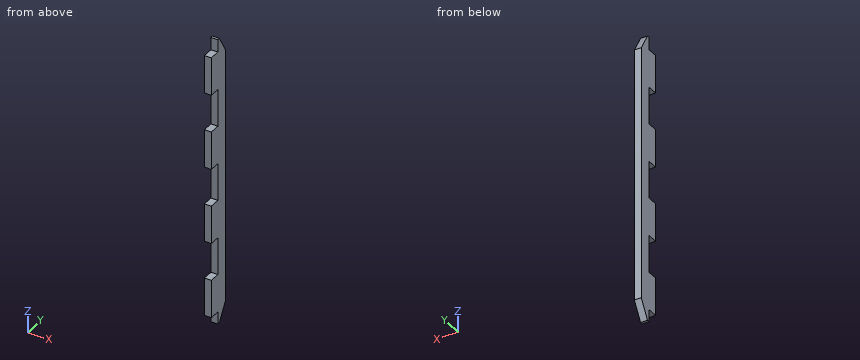
Autodesk Inventor part; units mm, degrees
ref_plane "YZ Plane" through (0, 0, 0) normal (1, 0, 0) x (0, 1, 0)
ref_plane "XZ Plane" through (0, 0, 0) normal (0, 1, 0) x (-1, 0, 0)
ref_plane "XY Plane" through (0, 0, 0) normal (0, 0, 1) x (1, 0, 0)
sketch "Sketch1" plane through (0, 0, 0) normal (1, 0, 0) x (0, 1, 0)
  line L0 (0, 0) -> (0, 115)
  line L1 (0, 115) -> (1, 115)
  line L2 (1, 115) -> (5, 108.0718)
  line L3 (5, 108.0718) -> (5, 6.9282)
  line L4 (5, 6.9282) -> (1, 0)
  line L5 (1, 0) -> (0, 0)
  line L6 (1, 115) -> (1, 0) construction
  dimension "d0" = 1
  dimension "d1" = 4
  dimension "d2" = 30
  dimension "d3" = 115
extrude "Extrusion1" add sketch "Sketch1" along normal blind 2.75
sketch "Sketch2" plane through (2.75, 0, 0) normal (1, 0, 0) x (0, 0, -1)
  line L0 (-115, 0) -> (0, 0)
  line L1 (-110, 0) -> (-94.85, 0)
  line L2 (-94.85, 0) -> (-94.85, -4.2)
  line L3 (-94.85, -4.2) -> (-110, -4.2)
  line L4 (-110, -4.2) -> (-110, 0)
  line L5 (-80, 0) -> (-64.85, 0)
  line L6 (-64.85, 0) -> (-64.85, -4.2)
  line L7 (-64.85, -4.2) -> (-80, -4.2)
  line L8 (-80, -4.2) -> (-80, 0)
  line L9 (-50, 0) -> (-34.85, 0)
  line L10 (-34.85, 0) -> (-34.85, -4.2)
  line L11 (-34.85, -4.2) -> (-50, -4.2)
  line L12 (-50, -4.2) -> (-50, 0)
  line L13 (-20, 0) -> (-4.85, 0)
  line L14 (-4.85, 0) -> (-4.85, -4.2)
  line L15 (-4.85, -4.2) -> (-20, -4.2)
  line L16 (-20, -4.2) -> (-20, 0)
  dimension "d6" = 15.15
  dimension "d7" = 15.15
  dimension "d8" = 15.15
  dimension "d9" = 15.15
  dimension "d10" = 4.2
  dimension "d11" = 5
  dimension "d12" = 30
  dimension "d13" = 30
  dimension "d14" = 30
extrude "Extrusion2" add sketch "Sketch2" against normal up to surface (2.75 mm away)
equation "\"d7\" = d6"
equation "\"d8\" = d6"
equation "\"d9\" = d6"
equation "\"d13\" = d12"
equation "\"d14\" = d12"
properties part number "TrayPanelH"
Geometry: final body of the model. Coordinates: model frame, mm. Round coordinates to 2 decimals unless told otherwise and drop trailing zeros. Write each loop counter-clockwise with the first axis right and the second up, starting at its lowest first coordinate (ties: lowest second). Pieces come first, ordered by that corner, then holes. Notation, with made-up numbers: (43, 11.25) -> (56, 11.25) arc R13 cw to (56, 24.25) -> close; hole circle Ø2 at (-10, 26.5). An arc over 180 degrees is marked (long way). Use CSV: the item, a comma, the result in double quotes. Start each with the question number.
Q1. Section C-C (z = 88). Return loops of the section in (x, y).
Q2. Section A-A (y = -3). Return loops of the section in (x, z), plus the area to 3 significant figures.
Q3. Section D-D (y = 2). Return loops of the section in (x, z), plus the area to 3 significant figures.
Q4. Section B-B (x = 1.5). Return loops of the section in (y, z).
Q5. Line query: L1, parallel to Z at x = 1.7, y = -0.5; L2, parallel to Y at x = 1.35, z = 54; L3, parallel to Z at x = 1.5, y = 4. Output: solid intervals per line, ascending.
Q6. First-contact query: pin 1 Ø1.4 at (x, y) = (1, -2) entering from +Z; pin 2 Ø0.8 at (x, z) = (2, 1.5) entering from -Y; pin 3 Ø1.4 at (x, y) = (1.5, -2.5) entering from -Z. Flat tips, straight axial feed; report the tip coordinate or a pass-through.
Result sheet:
1,outline,"(0, 0) -> (2.75, 0) -> (2.75, 5) -> (0, 5) -> close"
2,outline,"(0, 4.85) -> (2.75, 4.85) -> (2.75, 20) -> (0, 20) -> close; (0, 34.85) -> (2.75, 34.85) -> (2.75, 50) -> (0, 50) -> close; (0, 64.85) -> (2.75, 64.85) -> (2.75, 80) -> (0, 80) -> close; (0, 94.85) -> (2.75, 94.85) -> (2.75, 110) -> (0, 110) -> close"
2,area,"167 mm²"
3,outline,"(0, 1.73) -> (2.75, 1.73) -> (2.75, 113.27) -> (0, 113.27) -> close"
3,area,"307 mm²"
4,outline,"(-4.2, 4.85) -> (0, 4.85) -> (0, 0) -> (1, 0) -> (5, 6.93) -> (5, 108.07) -> (1, 115) -> (0, 115) -> (0, 110) -> (-4.2, 110) -> (-4.2, 94.85) -> (0, 94.85) -> (0, 80) -> (-4.2, 80) -> (-4.2, 64.85) -> (0, 64.85) -> (0, 50) -> (-4.2, 50) -> (-4.2, 34.85) -> (0, 34.85) -> (0, 20) -> (-4.2, 20) -> close"
5,L1,"4.85 to 20, 34.85 to 50, 64.85 to 80, 94.85 to 110"
5,L2,"0 to 5"
5,L3,"5.2 to 109.8"
6,pin 1,"z = 110"
6,pin 2,"y = 0"
6,pin 3,"z = 4.85"
